from build123d import *

# Parameters (mm, degrees)
F0_W     = 57.9882
F0_H     = 38.5318
F1_DEPTH = 10.033
F2_W     = 38.6842
F2_H     = 38.5318
F3_DEPTH = 9.652
F4_W     = 18.7452
F4_H     = 18.7452
F5_DEPTH = 9.652
F6_W     = 19.939
F6_H     = 38.5318
F7_DEPTH = 9.652


with BuildPart() as f1:
    # F0 (on Top) → F1 (new body)
    with BuildSketch(Plane.XY):
        Rectangle(F0_W, F0_H)
    extrude(amount=F1_DEPTH)

    # F2 (on face) → F3 (join)
    with BuildSketch(Plane.XY.offset(10.033)):
        with Locations((-9.652, 0)):
            Rectangle(F2_W, F2_H)
    extrude(amount=F3_DEPTH)

    # F4 (on face) → F5 (cut)
    with BuildSketch(Plane.XY.offset(19.685)):
        with Locations((0.3175, -0.2667)):
            Rectangle(F4_W, F4_H)
    extrude(amount=-F5_DEPTH, mode=Mode.SUBTRACT)

    # F6 (on face) → F7 (join)
    with BuildSketch(Plane.XY.offset(19.685)):
        with Locations((-19.0246, 0)):
            Rectangle(F6_W, F6_H)
    extrude(amount=F7_DEPTH)


solid = f1.part
For this review, take the finished solid that the model builds, in its own axes (mm). A direction names the side the tool comes from. Coordinates: 2 decimals unless noted, no trailing zeros. Loops run counter-clockwise (first coordinate to the right, second up) from the corner with the lowest first, then second, coordinate; pieces in that order, holes last. Notation, with made-up numbers: (49.25, 86.25) - (87.25, 86.25) arc R9 cw to (87.25, 97.25) - close; hole circle Ø7 at (7.25, 72.25). An arc over 180 degrees is marked (long way). Return JSON: item names as keys, results as strings.
Item 1: Take a section at C-C (x = 22). Give the boundary of the cut face in (y, z).
Determined:
{"outline": "(-19.27, 0) - (19.27, 0) - (19.27, 10.03) - (-19.27, 10.03) - close"}
Item 2: Insertion check: pin 1 (5 mm diameter, centred on x = 19, y = 7, fed in from +Z); pin 2 (10.5 mm diameter, centred on y = 12, z = 16, fed in from +X); pin 3 (3 mm diameter, centred on x = 1.5, y = -14, fed in from +Z) (3 decimals). Each pin has a flat end and moves straight along its axis. Give the tip position at first contact, or say it passes through.
Determined:
{"pin 1": "stops at z = 10.03", "pin 2": "stops at x = 9.69", "pin 3": "stops at z = 19.685"}
Item 3: Take a section at B-B (z = 14). Give the boundary of the cut face in (x, y), then the cut area to 3 significant figures.
Determined:
{"outline": "(-28.99, -19.27) - (9.69, -19.27) - (9.69, -9.64) - (-9.06, -9.64) - (-9.06, 9.11) - (9.69, 9.11) - (9.69, 19.27) - (-28.99, 19.27) - close", "area": "1,140 mm2"}
Item 4: For faces 5 (the flat face through (0, -9.639, 15)), 6 (the flat face through (0, -14, 19.685)), 7 (the flat face through (-28.994, 0, 14)), list the 3-axis set-ups (+Z, -Z, +X, -X, +Y, -Y) from which the entire face can be reached by the end or side of a thin tool; tool diameter is ignored.
Determined:
{"face 5": "+Z, +X", "face 6": "+Z, +X, +Y, -Y", "face 7": "+Z, -Z, -X, +Y, -Y"}
Item 5: Take a section at A-A (y = 16). Give the boundary of the cut face in (x, z) (3 decimals).
Determined:
{"outline": "(-28.994, 0) - (28.994, 0) - (28.994, 10.033) - (9.69, 10.033) - (9.69, 19.685) - (-9.055, 19.685) - (-9.055, 29.337) - (-28.994, 29.337) - close"}
Item 6: Mouldability with a two-part tool opening along Y and no side actions: class faces 1 (the flat face through (-19, 0, 29.337)), 2 (the flat face through (0, 9.106, 15)), 3 (the flat face through (14, 0, 10.033)), 4 (the flat face through (-7, -19.266, 11)) as pulls with the +Y half, pulls with the -Y half, needs draft (parallel to the pull), parting line crosses it, or undercut.
Determined:
{"face 1": "needs draft", "face 2": "undercut", "face 3": "undercut", "face 4": "pulls with the -Y half"}
Item 7: Take a section at D-D (y = 1). Give the boundary of the cut face in (x, z), then the cut area to 3 significant figures.
Determined:
{"outline": "(-28.99, 0) - (28.99, 0) - (28.99, 10.03) - (-9.06, 10.03) - (-9.06, 29.34) - (-28.99, 29.34) - close", "area": "967 mm2"}
Item 8: For line 1 (X direction, y = -1.5, z = 27.5); line 2 (Z direction, x = 13.5, y = 0); line 3 (X direction, y = 16.5, z = 11), list the stretches that pass through material, from the lowest coordinate up.
Determined:
{"line 1": "x = -28.99 to -9.06", "line 2": "z = 0 to 10.03", "line 3": "x = -28.99 to 9.69"}
